Input: part model. Units: mm. Frame: model coordinates. Round coordinates to 2 decimals unless told otherwise and drop trailing zeros. Write each loop counter-clockwise with the first axis right and the second up, starting at its lowest first coordinate (ties: lowest second). Pieces come first, ordered by that corner, then holes. Notation, with made-up numbers: (0, 2) -> (52, 2) arc R18 ccw to (52, 35) -> close; hole circle Ø3 at (83, 8.5). An arc over 180 degrees is marked (long way). Use CSV: the item, a comma, the result in double quotes.
```python
from build123d import *

# Parameters (mm, degrees)
SKETCH1_W                                   = 30
SKETCH1_H                                   = 70
EXTRUDE1_DEPTH                              = 2
CSK_FOR_FLAT_HEAD_MACHINE_SCREW1_AT_2_COUNT = 2
CSK_FOR_FLAT_HEAD_MACHINE_SCREW1_AT_2_PITCH = 50


with BuildPart() as part:
    # Sketch1 → Extrude1 (new body)
    with BuildSketch(Plane.XY):
        with Locations((15, 35)):
            Rectangle(SKETCH1_W, SKETCH1_H)
        with BuildLine():
            Line((12, 50), (18, 50))
            ThreePointArc((18, 50), (19.414213562, 49.414213562), (20, 48))
            Line((20, 48), (20, 22))
            ThreePointArc((20, 22), (19.414213562, 20.585786438), (18, 20))
            Line((18, 20), (12, 20))
            ThreePointArc((12, 20), (10.585786438, 20.585786438), (10, 22))
            Line((10, 22), (10, 48))
            ThreePointArc((10, 48), (10.585786438, 49.414213562), (12, 50))
        make_face(mode=Mode.SUBTRACT)
    extrude(amount=-EXTRUDE1_DEPTH)

    # Sketch2 → CSK for  Flat Head Machine Screw1 (revolve, cut)
    with BuildSketch(Plane(origin=(15, 60, 0), x_dir=(0, -1, 0), z_dir=(1, 0, 0))):
        Polygon((0, 0), (0, 2), (1.2, 2), (1.2, 1), (2.2, 0), align=None)
    csk_for_flat_head_machine_screw1 = revolve(axis=Axis((15, 60, 6.35), (0, 0, -1)), mode=Mode.SUBTRACT)

    # CSK for  Flat Head Machine Screw1 at 2: CSK for  Flat Head Machine Screw1 ×2
    with Locations(*[(0, -i * CSK_FOR_FLAT_HEAD_MACHINE_SCREW1_AT_2_PITCH, 0) for i in range(1, CSK_FOR_FLAT_HEAD_MACHINE_SCREW1_AT_2_COUNT)]):
        add(csk_for_flat_head_machine_screw1, mode=Mode.SUBTRACT)


solid = part.part
```
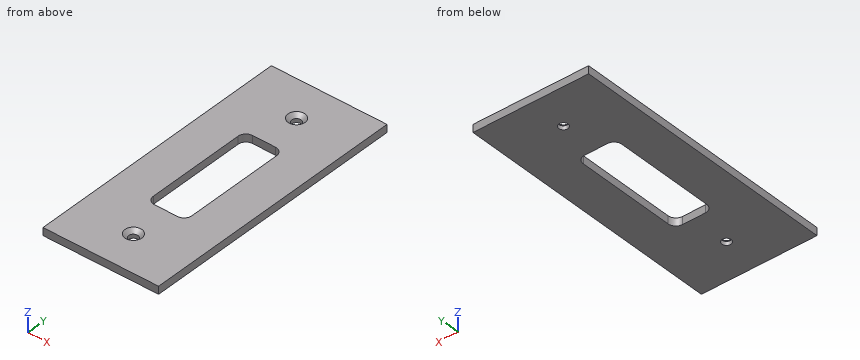
Item 1: Section query A-A on y = 31.5. Return the cut outline in (x, z), plus the area to 3 significant figures.
Worked answers:
outline,"(0, -2) -> (10, -2) -> (10, 0) -> (0, 0) -> close; (20, -2) -> (30, -2) -> (30, 0) -> (20, 0) -> close"
area,"40.0 mm²"
Item 2: Section query D-D on y = 10. Return the cut outline in (x, z), plus the area to 3 significant figures.
Worked answers:
outline,"(0, -2) -> (13.8, -2) -> (13.8, -1) -> (12.8, 0) -> (0, 0) -> close; (16.2, -2) -> (30, -2) -> (30, 0) -> (17.2, 0) -> (16.2, -1) -> close"
area,"54.2 mm²"
Item 3: Section query B-B on z = -0.55. Return the cut outline in (x, y).
Worked answers:
outline,"(0, 0) -> (30, 0) -> (30, 70) -> (0, 70) -> close; hole (10, 22) arc R2 ccw to (12, 20) -> (18, 20) arc R2 ccw to (20, 22) -> (20, 48) arc R2 ccw to (18, 50) -> (12, 50) arc R2 ccw to (10, 48) -> close; hole circle Ø3.3 at (15, 10); hole circle Ø3.3 at (15, 60)"
Item 4: Section query C-C on x = 15. Return the cut outline in (y, z).
Worked answers:
outline,"(0, -2) -> (8.8, -2) -> (8.8, -1) -> (7.8, 0) -> (0, 0) -> close; (11.2, -2) -> (20, -2) -> (20, 0) -> (12.2, 0) -> (11.2, -1) -> close; (50, -2) -> (58.8, -2) -> (58.8, -1) -> (57.8, 0) -> (50, 0) -> close; (61.2, -2) -> (70, -2) -> (70, 0) -> (62.2, 0) -> (61.2, -1) -> close"
Item 5: First-contact query: pin 1 Ø3 at (x, y) = (15, 60) entering from +Z. Flat tip, straight axial feed; report the tip coordinate or a pass-through.
Worked answers:
pin 1,"stops at z = -0.7"
Item 6: Line query: line 1 (Y direction, x = 15, z = -1.3); line 2 (X direction, y = 38, z = -1.8); line 3 (X direction, y = 60, z = -1.2). Output: solid intervals per line, ascending.
Worked answers:
line 1,"y = 0 to 8.8, 11.2 to 20, 50 to 58.8, 61.2 to 70"
line 2,"x = 0 to 10, 20 to 30"
line 3,"x = 0 to 13.8, 16.2 to 30"
